Autodesk Inventor part; units mm, degrees
ref_plane "YZ Plane" through (0, 0, 0) normal (1, 0, 0) x (0, 1, 0)
ref_plane "XZ Plane" through (0, 0, 0) normal (0, 1, 0) x (-1, 0, 0)
ref_plane "XY Plane" through (0, 0, 0) normal (0, 0, 1) x (1, 0, 0)
sketch "Boceto1" plane through (0, 0, 0) normal (0, 1, 0) x (-1, 0, 0)
  circle A0 centre (0, 0) radius 32.5
  line L0 (0, -22.5) -> (16, -22.5)
  line L1 (0, -22.5) -> (-16, -22.5)
  line L2 (-22.5, 0) -> (-22.5, -16)
  line L3 (-22.5, 0) -> (-22.5, 16)
  line L4 (0, 22.5) -> (16, 22.5)
  line L5 (0, 22.5) -> (-16, 22.5)
  line L6 (-16, 22.5) -> (-22.5, 16)
  line L7 (-22.5, -16) -> (-16, -22.5)
  line L8 (22.5, 0) -> (22.5, 16)
  line L9 (22.5, 0) -> (22.5, -16)
  line L10 (22.5, -16) -> (16, -22.5)
  line L11 (16, 22.5) -> (22.5, 16)
extrude "Extrusión1" add sketch "Boceto1" along normal blind 40
sketch "Boceto14" plane through (0, 0, 0) normal (0, -1, 0) x (1, 0, 0)
  line L0 (-16, 28.2887) -> (16, 28.2887)
  arc A0 (16, 28.2887) -> (-16, 28.2887) centre (0, 0) ccw
  point P0 (16, 22.5)
  point P1 (-16, 22.5)
extrude "Extrusión10" cut sketch "Boceto14" against normal blind 40
sketch "Boceto15" plane through (-22.5, 0, 16) normal (1, 0, 0) x (0, 0, -1)
  circle A0 centre (8, 8) radius 1.5
  circle A1 centre (24, 8) radius 1.5
  point P0 (16, 0)
  point P1 (0, 0)
  dimension "d80" = 3
  dimension "d81" = 3
extrude "Extrusión11" cut sketch "Boceto15" against normal mid plane 200
sketch "Boceto16" plane through (16, 0, 22.5) normal (0, 0, -1) x (-1, 0, 0)
  line L0 (-6.5, 0) -> (0, 0)
  circle A0 centre (8, 8) radius 1.5
  circle A1 centre (24, 8) radius 1.5
  point P0 (16, 0)
  dimension "d88" = 3
  dimension "d89" = 3
extrude "Extrusión12" cut sketch "Boceto16" along normal mid plane 200
sketch "Boceto17" plane through (16, 0, 22.5) normal (0, 0, -1) x (-1, 0, 0)
  circle A0 centre (8, 32) radius 1.5
  circle A1 centre (24, 32) radius 1.5
  point P0 (16, 0)
  point P1 (0, 40)
  dimension "d95" = 3
  dimension "d96" = 3
extrude "Extrusión13" cut sketch "Boceto17" against normal blind 200
properties part number "brazo_articulado_2" material "Plástico ABS"
The listing builds one solid part. Answer for the finished solid, in the listing's coordinates (mm). A direction names the side the tool comes from. Give positions to 0.01 mm unless a question says otherwise; leave off trailing zeros. Loops run counter-clockwise (first coordinate to the right, second up) from the corner with the lowest first, then second, coordinate; pieces in that order, holes last. Notation, with made-up numbers: M -23.5,22 L -6.5,22 A19 cw -6.5,58 Z; hole C 46,64 d7. An arc over 180 degrees is marked long. One line per item, written item: value.
1. For a pull along X with two mould halves and no side action, classify faces 4 (the face through (0, 20, -22.5)), 5 (the face through (-1.19, 19.72, -32.48)), 6 (the face through (27.237, 7.425, 6.614)) as pulls with the +X half, pulls with the -X half, needs draft (parallel to the pull), parting line crosses it, or undercut.
Found:
face 4: undercut
face 5: parting line crosses it
face 6: needs draft
2. Section D-D on x = 0 is taken. Determine the outline of the cut face in (y, z), plus the area to 3 significant figures.
Found:
outline: M 0,-32.5 L 40,-32.5 L 40,-22.5 L 0,-22.5 Z; M 0,22.5 L 40,22.5 L 40,28.29 L 0,28.29 Z
area: 632 mm^2
3. Each of these flat-tipped pins is pushed along its axis until it touches: P1, Ø3.5, axis at y = 8, z = 8, coming from the -X side; P2, Ø10, axis at y = 20.5, z = 1, coming from the +X side; P3, Ø8, axis at y = 17, z = 20, coming from the -X side; P4, Ø5, axis at x = -8, y = 8, coming from the +Z side. Where does it stop, or does it pass through?
Found:
P1: x = -31.89
P2: x = 32.5
P3: x = -28.29
P4: z = 28.29
4. For faces 1 (the face through (19.3, 19.7, -19.2)), 2 (the face through (-7.675, 30.536, 25.354)), 3 (the face through (3, 0, -24)), determine the directions among +Z, -Z, +X, -X, +Y, -Y from which every point of the face is accessible in a straight line to the end or side of a thin tool.
Found:
face 1: +Y, -Y
face 2: +Z
face 3: +Z, -Z, +X, -X, -Y
5. Find the intervals of material crossed by probe 1 along Y at (x, z) = (8, 26); probe 2 along X at (y, z) = (16, 0); probe 3 along X at (y, z) = (7.5, 23.5), in increasing order.
Found:
probe 1: 0 to 6.5, 9.5 to 30.5, 33.5 to 40
probe 2: -32.5 to -22.5, 22.5 to 32.5
probe 3: -22.45 to -9.41, -6.59 to 6.59, 9.41 to 22.45
6. Section C-C on y = 4 is taken. Determine the outline of the cut face in (x, z).
Found:
outline: M -16,28.29 A32.5 ccw long 16,28.29 Z; hole M -22.5,-16 L -16,-22.5 L 16,-22.5 L 22.5,-16 L 22.5,16 L 16,22.5 L -16,22.5 L -22.5,16 Z
7. Section A-A on z = 8 is taken. Determine the outline of the cut face in (x, y).
Found:
outline: M -31.5,0 L -22.5,0 L -22.5,6.5 L -31.5,6.5 Z; M -31.5,9.5 L -22.5,9.5 L -22.5,40 L -31.5,40 Z; M 22.5,0 L 31.5,0 L 31.5,6.5 L 22.5,6.5 Z; M 22.5,9.5 L 31.5,9.5 L 31.5,40 L 22.5,40 Z
8. Section B-B on x = -8 is taken. Determine the outline of the cut face in (y, z), plus the area to 3 significant figures.
Found:
outline: M 0,-31.5 L 6.5,-31.5 L 6.5,-22.5 L 0,-22.5 Z; M 0,22.5 L 6.5,22.5 L 6.5,28.29 L 0,28.29 Z; M 9.5,-31.5 L 40,-31.5 L 40,-22.5 L 9.5,-22.5 Z; M 9.5,22.5 L 30.5,22.5 L 30.5,28.29 L 9.5,28.29 Z; M 33.5,22.5 L 40,22.5 L 40,28.29 L 33.5,28.29 Z
area: 530 mm^2
